from build123d import *

# Parameters (mm, degrees)
FILLET1_R          = 2
SKETCH2_R          = 3
CUT_EXTRUDE1_DEPTH = 3.2


with BuildPart() as part:
    # Sketch1 → Revolve1 (revolve)
    with BuildSketch(Plane.XY, mode=Mode.PRIVATE) as revolve1_sk:
        Polygon((0, 0), (8, 0), (8, -4), (4, -8), (4, -13.535898385), (6, -17), (6, -20), (0, -20), align=None)
    revolve(revolve1_sk.sketch.rotate(Axis((0, 48.586008243, 0), (0, -1, 0)), 90), axis=Axis((0, 48.586008243, 0), (0, -1, 0)))

    # Fillet1
    fillet1_edges = [part.edges().sort_by_distance(p)[0] for p in [
        (0, -20, -6),
        (0, -17, -6),
        (0, -13.535898385, -4),
        (0, -8, -4),
        (0, -4, -8),
    ]]
    fillet(fillet1_edges, radius=FILLET1_R)

    # Sketch2 → Cut-Extrude1 (cut)
    with BuildSketch(Plane(origin=(0, 0, 0), x_dir=(1, 0, 0), z_dir=(0, 1, 0))):
        with Locations(Location((0, 0, 0), (0, 0, 270))):
            Circle(SKETCH2_R)
    extrude(amount=-CUT_EXTRUDE1_DEPTH, mode=Mode.SUBTRACT)


solid = part.part
Geometry: final body of the model. Coordinates: model frame, mm. A direction names the side the tool comes from. Coordinates: 2 decimals unless noted, no trailing zeros. Write each loop counter-clockwise with the first axis right and the second up, starting at its lowest first coordinate (ties: lowest second). Pieces come first, ordered by that corner, then holes. Notation, with made-up numbers: (18.5, 23.5) - (43.5, 23.5) arc R11 cw to (43.5, 41.5) - close; hole circle Ø8 at (-25, 20.5). An arc over 180 degrees is marked (long way). Return JSON: item names as keys, results as strings.
Item 1: Reachability of faces 1 (the face through (3.549, -10.943, 1.846)), 2 (the face through (7.81, -1.61, -1.73)), 3 (the face through (-1.802, -17.771, 5.723)) from +Z, -Z, +X, -X, +Y, -Y: full face, straight path, thin tool, end or side. Return the list, or none.
Completed:
{"face 1": "none", "face 2": "+Y, -Y", "face 3": "-Y"}
Item 2: Section query A-A (y = -1.25). Output: boundary loops of the cut face in (x, z), and give its area (3 significant figures).
Completed:
{"outline": "circle Ø16 at (0, 0); hole circle Ø6 at (0, 0)", "area": "173 mm2"}
Item 3: Section query C-C (y = -18.25). Output: boundary loops of the cut face in (x, z), and give its area (3 significant figures).
Completed:
{"outline": "circle Ø11.97 at (0, 0)", "area": "113 mm2"}
Item 4: Pin query (flat end, axial travel): pin 1 Ø6 at (x, y) = (1, -14.5) entering from +Z; pin 2 Ø3 at (x, z) = (0.5, -1) entering from +Y; pin 3 Ø4 at (x, y) = (-3.5, -11.5) entering from -Z. Return the tip coordinate at first contact, or that it passes through.
Completed:
{"pin 1": "stops at z = 5.99", "pin 2": "stops at y = -3.2", "pin 3": "stops at z = -3.71"}
Item 5: Section query B-B (y = -6.25). Output: boundary loops of the cut face in (x, z), and give its area (3 significant figures).
Completed:
{"outline": "circle Ø11.5 at (0, 0)", "area": "104 mm2"}
Item 6: Pull-direction query (Z, two-part tool) for faces 4 (the face through (0.9, -1.58, 2.86)), 5 (the face through (0, -3.2, 0)), 6 (the face through (-0.1, 0, -3.4)), 7 (the face through (-1.419, -7.277, 4.505)); classes: +Z half, -Z half, draft (parallel to the pull), parting line (faces both ways), or undercut.
Completed:
{"face 4": "undercut", "face 5": "undercut", "face 6": "draft", "face 7": "parting line"}
Item 7: Line query: L1, parallel to X at y = -2.15, z = 0; L2, parallel to Y at x = 5.5, z = 1.5; L3, parallel to Y at x = -0.5, z = -4.75. Output: solid intervals per line, ascending.
Completed:
{"L1": "x = -8 to -3, 3 to 8", "L2": "y = -19.05 to -16.48, -6.3 to 0", "L3": "y = -19.84 to -14.88, -7.22 to 0"}
